The listing builds one solid part. Answer for the finished solid, in the listing's coordinates (mm). A direction names the side the tool comes from. Give positions to 0.01 mm unless a question says otherwise; leave off trailing zeros. Write each loop counter-clockwise with the first axis right and the second up, starting at its lowest first coordinate (ties: lowest second). Pieces come first, ordered by that corner, then holes.
```python
from build123d import *

# Parameters (mm, degrees)
F1_R         = 7.5
F1_R_2       = 3.2691742077
F2_DEPTH     = 3
F3_W         = 3
F3_H         = 15
F4_DEPTH     = 15
F5_R         = 3.2691742077
F6_DEPTH     = 50.751
F7_T1_DEPTH  = 3
F7_T3_DEPTH  = 3
F7_T5_DEPTH  = 3
F7_T7_DEPTH  = 28
F7_T9_DEPTH  = 15.5
F7_T11_DEPTH = 28
F7_T13_DEPTH = 28
F7_T15_DEPTH = 15.5
F8_R         = 0.99999


# Not quite as in the source:
# - a fillet or chamfer that OpenCascade refuses, or shapes differently, is made with other operations: its cross-section is extruded or revolved along the edge and cut away or added
# - a fillet or chamfer is up to 0.001 mm smaller than in the source, because OpenCascade refuses the exact size


with BuildPart() as f2:
    # F1 (on Top) → F2 (new body)
    with BuildSketch(Plane.XY):
        Polygon((41, 15), (-41, 15), (-41, -15), (-9.75, -15), (9.75, -15), (41, -15), align=None)
        with BuildLine():
            ThreePointArc((-17.5600507895, -5.3635116598), (-34.7645626416, -4.8148148148), (-26, 10))
            Line((-26, 10), (-14.1678404338, 10))
            ThreePointArc((-14.1678404338, 10), (-11.1002435092, 8.1851851852), (-11.2138582101, 4.6227709191))
            Line((-11.2138582101, 4.6227709191), (-17.5600507895, -5.3635116598))
        make_face(mode=Mode.SUBTRACT)
        Circle(F1_R, mode=Mode.SUBTRACT)
        with BuildLine():
            ThreePointArc((17.5600507895, 5.3635116598), (34.7645626416, 4.8148148148), (26, -10))
            Line((26, -10), (14.1678404338, -10))
            ThreePointArc((14.1678404338, -10), (11.1002435092, -8.1851851852), (11.2138582101, -4.6227709191))
            Line((11.2138582101, -4.6227709191), (17.5600507895, 5.3635116598))
        make_face(mode=Mode.SUBTRACT)
        Polygon((9.75, -15), (-9.75, -15), (-9.75, -65), (-6.75, -65), (-6.75, -45), (-4.75, -45), (-4.75, -65), (4.75, -65), (4.75, -45), (6.75, -45), (6.75, -65), (9.75, -65), align=None)
        with Locations((0, -57.5)):
            Circle(F1_R_2, mode=Mode.SUBTRACT)
    extrude(amount=F2_DEPTH)

    # F3 (on face) → F4 (join)
    with BuildSketch(Plane(origin=(0, 0, 0), x_dir=(1, 0, 0), z_dir=(0, 0, -1))):
        with Locations((8.25, 57.5)):
            Rectangle(F3_W, F3_H)
        with Locations((-8.25, 57.5)):
            Rectangle(F3_W, F3_H)
    extrude(amount=F4_DEPTH)

    # F5 (on face) → F6 (cut, through all)
    with BuildSketch(Plane.YZ.offset(9.75)):
        with Locations((-57.5, -6.75)):
            Circle(F5_R)
    extrude(amount=-F6_DEPTH, mode=Mode.SUBTRACT)

    # F7: fillet of radius 5 on 16 edges, made by hand

    # F7_s2 → F7_t1 (join)
    with BuildSketch(Plane.XY):
        with BuildLine():
            ThreePointArc((-14.75, -15), (-11.2144660941, -16.4644660941), (-9.75, -20))
            Line((-9.75, -20), (-9.75, -15))
            Line((-9.75, -15), (-14.75, -15))
        make_face()
        with BuildLine():
            ThreePointArc((14.75, -15), (11.2144660941, -16.4644660941), (9.75, -20))
            Line((9.75, -20), (9.75, -15))
            Line((9.75, -15), (14.75, -15))
        make_face()
    extrude(amount=F7_T1_DEPTH)

    # F7_s4 → F7_t3 (join)
    with BuildSketch(Plane.YZ.offset(6.75)):
        with BuildLine():
            ThreePointArc((-45, 0), (-48.5355339059, -1.4644660941), (-50, -5))
            Line((-50, -5), (-50, 0))
            Line((-50, 0), (-45, 0))
        make_face()
    extrude(amount=F7_T3_DEPTH)

    # F7_s6 → F7_t5 (join)
    with BuildSketch(Plane.YZ.offset(-9.75)):
        with BuildLine():
            ThreePointArc((-45, 0), (-48.5355339059, -1.4644660941), (-50, -5))
            Line((-50, -5), (-50, 0))
            Line((-50, 0), (-45, 0))
        make_face()
    extrude(amount=F7_T5_DEPTH)

    # F7_s8 → F7_t7 (cut)
    with BuildSketch(Plane.XY.offset(-12.5)):
        with BuildLine():
            ThreePointArc((-36, 15), (-39.5355339059, 13.5355339059), (-41, 10))
            Line((-41, 10), (-41, 15))
            Line((-41, 15), (-36, 15))
        make_face()
        with BuildLine():
            ThreePointArc((36, 15), (39.5355339059, 13.5355339059), (41, 10))
            Line((41, 10), (41, 15))
            Line((41, 15), (36, 15))
        make_face()
        with BuildLine():
            ThreePointArc((41, -10), (39.5355339059, -13.5355339059), (36, -15))
            Line((36, -15), (41, -15))
            Line((41, -15), (41, -10))
        make_face()
        with BuildLine():
            ThreePointArc((-41, -10), (-39.5355339059, -13.5355339059), (-36, -15))
            Line((-36, -15), (-41, -15))
            Line((-41, -15), (-41, -10))
        make_face()
        with BuildLine():
            ThreePointArc((4.75, -60), (3.2855339059, -63.5355339059), (-0.25, -65))
            Line((-0.25, -65), (4.75, -65))
            Line((4.75, -65), (4.75, -60))
        make_face()
        with BuildLine():
            ThreePointArc((0.25, -65), (-3.2855339059, -63.5355339059), (-4.75, -60))
            Line((-4.75, -60), (-4.75, -65))
            Line((-4.75, -65), (0.25, -65))
        make_face()
    extrude(amount=F7_T7_DEPTH, mode=Mode.SUBTRACT)

    # F7_s10 → F7_t9 (cut)
    with BuildSketch(Plane.YZ.offset(-22.25)):
        with BuildLine():
            ThreePointArc((-60, 3), (-63.5355339059, 1.5355339059), (-65, -2))
            Line((-65, -2), (-65, 3))
            Line((-65, 3), (-60, 3))
        make_face()
    extrude(amount=F7_T9_DEPTH, mode=Mode.SUBTRACT)

    # F7_s12 → F7_t11 (cut)
    with BuildSketch(Plane.YZ.offset(-22.25)):
        with BuildLine():
            ThreePointArc((-50, -10), (-51.4644660941, -13.5355339059), (-55, -15))
            Line((-55, -15), (-50, -15))
            Line((-50, -15), (-50, -10))
        make_face()
        with BuildLine():
            ThreePointArc((-65, -10), (-63.5355339059, -13.5355339059), (-60, -15))
            Line((-60, -15), (-65, -15))
            Line((-65, -15), (-65, -10))
        make_face()
    extrude(amount=F7_T11_DEPTH, mode=Mode.SUBTRACT)

    # F7_s14 → F7_t13 (cut)
    with BuildSketch(Plane.YZ.offset(-5.75)):
        with BuildLine():
            ThreePointArc((-55, -15), (-51.4644660941, -13.5355339059), (-50, -10))
            Line((-50, -10), (-50, -15))
            Line((-50, -15), (-55, -15))
        make_face()
        with BuildLine():
            ThreePointArc((-65, -10), (-63.5355339059, -13.5355339059), (-60, -15))
            Line((-60, -15), (-65, -15))
            Line((-65, -15), (-65, -10))
        make_face()
    extrude(amount=F7_T13_DEPTH, mode=Mode.SUBTRACT)

    # F7_s16 → F7_t15 (cut)
    with BuildSketch(Plane.YZ.offset(6.75)):
        with BuildLine():
            ThreePointArc((-60, 3), (-63.5355339059, 1.5355339059), (-65, -2))
            Line((-65, -2), (-65, 3))
            Line((-65, 3), (-60, 3))
        make_face()
    extrude(amount=F7_T15_DEPTH, mode=Mode.SUBTRACT)

    # F8 (radius 1 in the source; OpenCascade refuses exactly that, so slightly less here)
    f8_edges = [f2.edges().sort_by_distance(p)[0] for p in [
        (4.75, -45, 1.5),
        (6.75, -45, 1.5),
        (-4.75, -45, 1.5),
        (-6.75, -45, 1.5),
    ]]
    fillet(f8_edges, radius=F8_R)


solid = f2.part
```
Item 1: A cutting plane is placed at D-D, the plane z = -13.5. Give the vertices of the cut face in (x, y), plus the area to 3 significant figures.
Conclusion:
outline: (-9.75, -63.57) - (-6.75, -63.57) - (-6.75, -51.43) - (-9.75, -51.43) - close; (6.75, -63.57) - (9.75, -63.57) - (9.75, -51.43) - (6.75, -51.43) - close
area: 72.8 mm2
Item 2: A cutting plane is placed at C-C, the plane z = -6.75. Give the vertices of the cut face in (x, y).
Conclusion:
outline: (-9.75, -65) - (-6.75, -65) - (-6.75, -60.77) - (-9.75, -60.77) - close; (-9.75, -54.23) - (-6.75, -54.23) - (-6.75, -50) - (-9.75, -50) - close; (6.75, -65) - (9.75, -65) - (9.75, -60.77) - (6.75, -60.77) - close; (6.75, -54.23) - (9.75, -54.23) - (9.75, -50) - (6.75, -50) - close
Item 3: A cutting plane is placed at B-B, the plane y = -57.5. Give the vertices of the cut face in (x, z), plus the area to 3 significant figures.
Conclusion:
outline: (-9.75, -15) - (-6.75, -15) - (-6.75, -10.02) - (-9.75, -10.02) - close; (-9.75, -3.48) - (-6.75, -3.48) - (-6.75, 3) - (-9.75, 3) - close; (-4.75, 0) - (-3.27, 0) - (-3.27, 3) - (-4.75, 3) - close; (3.27, 0) - (4.75, 0) - (4.75, 3) - (3.27, 3) - close; (6.75, -15) - (9.75, -15) - (9.75, -10.02) - (6.75, -10.02) - close; (6.75, -3.48) - (9.75, -3.48) - (9.75, 3) - (6.75, 3) - close
area: 77.7 mm2
Item 4: A cutting plane is placed at A-A, the plane x = 32. Give the vertices of the cut face in (y, z), plus the area to 3 significant figures.
Conclusion:
outline: (-15, 0) - (-8, 0) - (-8, 3) - (-15, 3) - close; (8, 0) - (15, 0) - (15, 3) - (8, 3) - close
area: 42.0 mm2
Item 5: Determine the mould class of faces 1 (the face through (-8.229, -60.766, -6.606)), 2 (the face through (8, -52, -14)), 3 (the face through (-41, 0, 1)) for opening direction Z: pulls with the +Z half, pulls with the -Z half, needs draft (parallel to the pull), parting line crosses it, or undercut.
Conclusion:
face 1: undercut
face 2: pulls with the -Z half
face 3: needs draft
Item 6: Consider probe 1 along X at (y, z) = (-53, -12.5); probe 2 along Y at (x, z) = (-26, 1.45); probe 3 along Z at (x, y) = (4.5, 12.5). Determine where each line is inside the solid, lowest interval first.
Conclusion:
probe 1: x = -9.75 to -6.75, 6.75 to 9.75
probe 2: y = -15 to -10, 10 to 15
probe 3: z = 0 to 3
Item 7: Each of these flat-tipped pins is pushed along its axis until it touches: P1, Ø8, axis at x = -11.5, z = -12.5, coming from the +Y side; P2, Ø16, axis at x = 26, y = 0, coming from the +Z side; P3, Ø9, axis at y = -58, z = -4, coming from the -X side; P4, Ø3.5, axis at x = -19, z = 1, coming from the -Y side. Where does it stop, or does it pass through?
Conclusion:
P1: stops at y = -50
P2: passes through
P3: stops at x = -9.75
P4: stops at y = -15
Item 8: Which of the six approach directions +Z, -Z, +X, -X, +Y, -Y give full straight-line access (tool end or side, diameter ignored) to faces 4 (the face through (-3.34, -63.48, 1.48)), 5 (the face through (20, -10, 1)), 6 (the face through (8, -50, -7))?
Conclusion:
face 4: +Z, -Z, -Y
face 5: +Z, -Z
face 6: -Z, +X, -X, +Y
